Design review of the part shown in the three views and the two pictorial views. Dimensions are in mm from the part's minimum x, y and z. Give positions to 0.01 mm unless a question says otherwise; leave off trailing zeros. Order: outer loops, then holes, each group sorted by start corner. A loop starts at its lowest first (then second) coordinate and runs counter-clockwise, first axis right, second up. Notation, with made-up numbers: (20, 67) - (55, 67) arc R20 cw to (55, 79) - close; hole circle Ø8 at (84.25, -0.75). An arc over 180 degrees is marked (long way). Put each result on its own line as item: value.
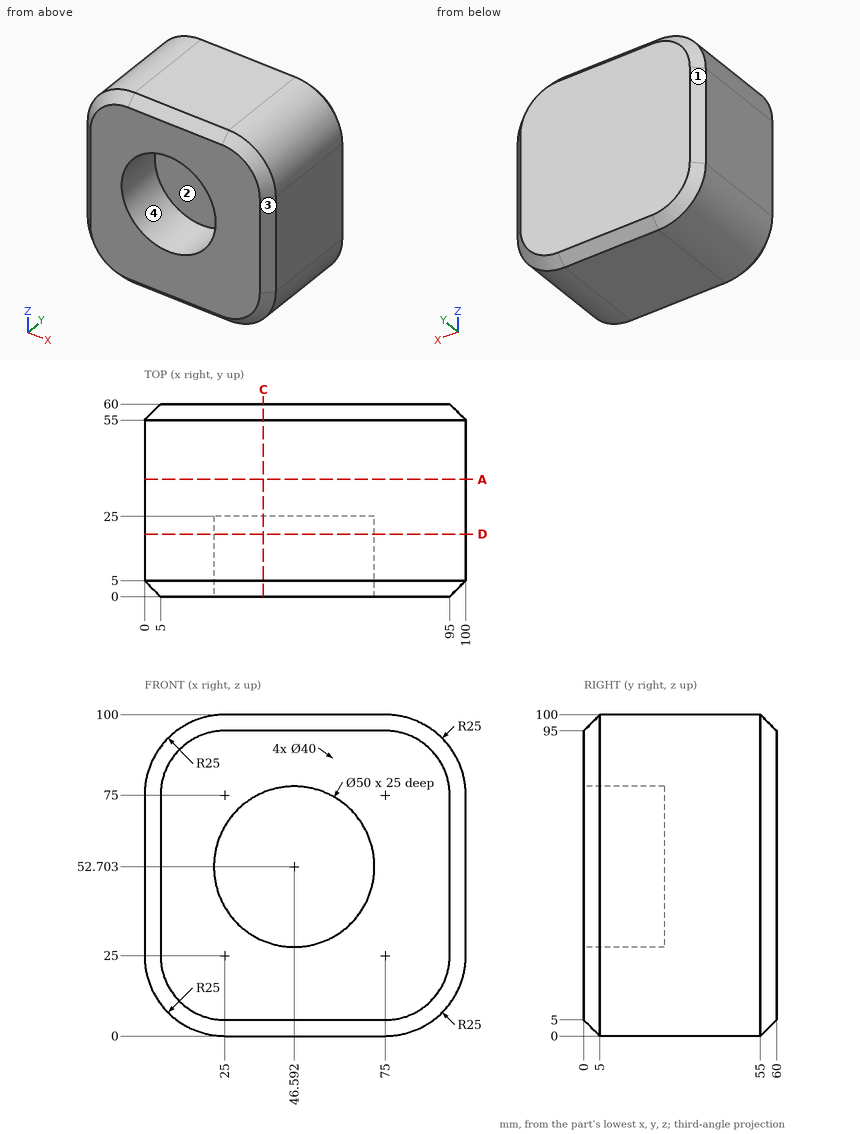
(1) Wall thickness on L1, parallel to X at y = 30, z = 90; L2, parallel to Y at x = 45.5, z = 54; L3, parallel to X at y = 6, z = 46.5 (1 decimal): over which ranges is each line inside the solid? List them lowest first.
The answers:
L1: 5 to 95
L2: 25 to 60
L3: 0 to 22.4, 70.8 to 100
(2) Take a section at D-D, the plane y = 19.5. Write out the cut boundary in (x, z).
The answers:
outline: (0, 25) arc R25 ccw to (25, 0) - (75, 0) arc R25 ccw to (100, 25) - (100, 75) arc R25 ccw to (75, 100) - (25, 100) arc R25 ccw to (0, 75) - close; hole circle Ø50 at (46.59, 52.7)
(3) The part is to be moulded in two halves that separate along X. For the marked faces 1, 2, 3 and 4, say which applies: pulls with the +X half, pulls with the -X half, needs draft (parallel to the pull), parting line crosses it, or undercut.
The answers:
face 1: pulls with the -X half
face 2: undercut
face 3: pulls with the +X half
face 4: undercut
(4) Take a section at C-C, the plane x = 37. Write out the cut boundary in (y, z), then the cut area to 3 significant figures.
The answers:
outline: (0, 5) - (5, 0) - (55, 0) - (60, 5) - (60, 95) - (55, 100) - (5, 100) - (0, 95) - (0, 75.79) - (25, 75.79) - (25, 29.62) - (0, 29.62) - close
area: 4,800 mm^2
(5) Take a section at A-A, the plane y = 36.5. Write out the cut boundary in (x, z).
The answers:
outline: (0, 25) arc R25 ccw to (25, 0) - (75, 0) arc R25 ccw to (100, 25) - (100, 75) arc R25 ccw to (75, 100) - (25, 100) arc R25 ccw to (0, 75) - close
(6) Clearance check with flat-ended pins moving along their axes: pin 1 Ø6 at (x, z) = (46, 32.5) entering from -Y; pin 2 Ø4 at (x, y) = (12, 10) entering from -Z; pin 3 Ø6 at (x, y) = (81, 51) entering from +Z. State where each tip first meets the part, or that it passes through.
The answers:
pin 1: y = 25
pin 2: z = 2.55
pin 3: z = 99.82
